```python
from build123d import *

# Parameters (mm, degrees)
SKETCH1_W           = 120
SKETCH1_H           = 30
BOSS_EXTRUDE1_DEPTH = 3
SKETCH2_W           = 28.5
SKETCH2_H           = 30
SKETCH2_W_2         = 20.5
SKETCH2_H_2         = 20.5
BOSS_EXTRUDE2_DEPTH = 20
CHAMFER1_SIZE       = 3
CHAMFER2_SIZE       = 3
CUT_EXTRUDE1_DEPTH  = 20
SKETCH4_R           = 1.65
CUT_EXTRUDE2_DEPTH  = 40
CUT_EXTRUDE3_DEPTH  = 40
SKETCH6_W           = 45.75
SKETCH6_H           = 2
BOSS_EXTRUDE3_DEPTH = 17
CUT_EXTRUDE5_DEPTH  = 17
SKETCH8_R           = 3.302
CUT_EXTRUDE6_DEPTH  = 17
FILLET1_R           = 5


with BuildPart() as part:
    # Sketch1 → Boss-Extrude1 (new body)
    with BuildSketch(Plane(origin=(0, 0, 0), x_dir=(1, 0, 0), z_dir=(0, 1, 0))):
        Rectangle(SKETCH1_W, SKETCH1_H)
    extrude(amount=BOSS_EXTRUDE1_DEPTH)

    # Sketch2 → Boss-Extrude2 (add)
    with BuildSketch(Plane(origin=(0, 3, 0), x_dir=(1, 0, 0), z_dir=(0, 1, 0))):
        Rectangle(SKETCH2_W, SKETCH2_H)
        Rectangle(SKETCH2_W_2, SKETCH2_H_2, mode=Mode.SUBTRACT)
    extrude(amount=BOSS_EXTRUDE2_DEPTH)

    # Chamfer1
    chamfer1_edges = [part.edges().sort_by_distance(p)[0] for p in [
        (14.25, 13, 15),
        (14.25, 13, -15),
        (-14.25, 13, -15),
        (-14.25, 13, 15),
    ]]
    chamfer(chamfer1_edges, length=CHAMFER1_SIZE)

    # Chamfer2
    # the kernel refuses this chamfer: 3 mm, written as the material it takes off along each edge
    with BuildSketch(Plane(origin=(18.965048964, 23, -15), x_dir=(0, -0.9996219169112968, -0.02749587661058619), z_dir=(-1, 0, 0)), Plane(origin=(-18.965048964, 23, 15), x_dir=(0, -0.9996219169112968, 0.02749587661058619), z_dir=(1, 0, 0))) as chamfer2_piece_1:
        Polygon((CHAMFER2_SIZE * 0.999621916911, CHAMFER2_SIZE * 0.0274958766106), (-CHAMFER2_SIZE * 0.0274958766106, CHAMFER2_SIZE * 0.999621916911), (0, 0), align=None)
    extrude(amount=37.930097928, mode=Mode.SUBTRACT)
    with BuildSketch(Plane(origin=(14.25, 23, 19.715048964), x_dir=(0.02749587661058619, -0.9996219169112968, 0), z_dir=(0, 0, -1)), Plane(origin=(-14.25, 23, -19.715048964), x_dir=(-0.02749587661058619, -0.9996219169112968, 0), z_dir=(0, 0, 1))) as chamfer2_piece_2:
        Polygon((CHAMFER2_SIZE * 0.999621916911, CHAMFER2_SIZE * 0.0274958766106), (-CHAMFER2_SIZE * 0.0274958766106, CHAMFER2_SIZE * 0.999621916911), (0, 0), align=None)
    extrude(amount=39.430097928, mode=Mode.SUBTRACT)

    # Sketch3 → Cut-Extrude1 (cut)
    with BuildSketch(Plane(origin=(0, 3, 0), x_dir=(1, 0, 0), z_dir=(0, 1, 0))):
        Polygon((-11.25, 15), (-60, 8), (-60, 15), align=None)
        Polygon((-11.25, -15), (-60, -8), (-60, -15), align=None)
        Polygon((11.25, 15), (60, 15), (60, 8), align=None)
        Polygon((11.25, -15), (60, -15), (60, -8), align=None)
    extrude(amount=-CUT_EXTRUDE1_DEPTH, mode=Mode.SUBTRACT)

    # Sketch4 → Cut-Extrude2 (cut)
    with BuildSketch(Plane.XY.offset(15)):
        with Locations((0, 10.735706987)):
            Circle(SKETCH4_R)
    extrude(amount=-CUT_EXTRUDE2_DEPTH, mode=Mode.SUBTRACT)

    # Sketch5 → Cut-Extrude3 (cut)
    with BuildSketch(Plane(origin=(0, 3, 0), x_dir=(1, 0, 0), z_dir=(0, 1, 0))):
        with BuildLine():
            Line((-9, -1), (-5.916079783, -1))
            ThreePointArc((-5.916079783, -1), (-4.242640687, -4.242640687), (-1, -5.916079783))
            Line((-1, -5.916079783), (-1, -9))
            Line((-1, -9), (1, -9))
            Line((1, -9), (1, -5.916079783))
            ThreePointArc((1, -5.916079783), (4.242640687, -4.242640687), (5.916079783, -1))
            Line((5.916079783, -1), (9, -1))
            Line((9, -1), (9, 1))
            Line((9, 1), (5.916079783, 1))
            ThreePointArc((5.916079783, 1), (4.242640687, 4.242640687), (1, 5.916079783))
            Line((1, 5.916079783), (1, 9))
            Line((1, 9), (-1, 9))
            Line((-1, 9), (-1, 5.916079783))
            ThreePointArc((-1, 5.916079783), (-4.242640687, 4.242640687), (-5.916079783, 1))
            Line((-5.916079783, 1), (-9, 1))
            Line((-9, 1), (-9, -1))
        make_face()
    extrude(amount=-CUT_EXTRUDE3_DEPTH, mode=Mode.SUBTRACT)

    # Sketch6 → Boss-Extrude3 (add)
    with BuildSketch(Plane(origin=(0, 3, 0), x_dir=(1, 0, 0), z_dir=(0, 1, 0))):
        with Locations((-37.125, 0.087113991)):
            Rectangle(SKETCH6_W, SKETCH6_H)
        with Locations((37.125, 0.087113991)):
            Rectangle(SKETCH6_W, SKETCH6_H)
    extrude(amount=BOSS_EXTRUDE3_DEPTH)

    # Sketch7 → Cut-Extrude5 (cut)
    with BuildSketch(Plane.XY.offset(0.912886009)):
        Polygon((-14.25, 20), (-60, 3), (-66.007429388, 26.966086251), align=None)
        Polygon((14.25, 20), (60, 3), (71.057586423, 29.350453949), align=None)
    extrude(amount=-CUT_EXTRUDE5_DEPTH, mode=Mode.SUBTRACT)

    # Sketch8 → Cut-Extrude6 (cut)
    with BuildSketch(Plane.XY.offset(0.912886009)):
        with Locations((-29.25, 8.622465364)):
            Circle(SKETCH8_R)
        with Locations((29.25, 8.622465364)):
            Circle(SKETCH8_R)
    extrude(amount=-CUT_EXTRUDE6_DEPTH, mode=Mode.SUBTRACT)

    # Fillet1
    fillet1_edges = [part.edges().sort_by_distance(p)[0] for p in [
        (-60, 1.5, -8),
        (-60, 1.5, 8),
        (60, 1.5, -8),
        (60, 1.5, 8),
    ]]
    fillet(fillet1_edges, radius=FILLET1_R)


solid = part.part
```
Here's how the part is built. I have some questions about the finished solid (model axes, mm). A direction names the side the tool comes from. Round coordinates to 2 decimals unless told otherwise and drop trailing zeros. Order: outer loops, then holes, each group sorted by start corner. A loop starts at its lowest first (then second) coordinate and runs counter-clockwise, first axis right, second up. Notation, with made-up numbers: (17.5, -14.5) -> (55.5, -14.5) arc R21 ccw to (55.5, 2.5) -> close; hole circle Ø5 at (65, 56.5). An arc over 180 degrees is marked (long way). Use a Markdown table: item, result. Add a question column.
(1) Suppose I cut it at C-C, the plane x = -3.5. Please give me the cut outline in (y, z), and give its area (3 significant figures).
(2) I need wall thicknesses on line 1 along X through (y, z) = (10.5, -2.5); line 2 along Y through (x, z) = (0, 11.8); line 3 along Y through (x, z) = (-19.5, -5.5). Which ranges of each line are inside material? Lowest first, please.
(3) Suppose I cut it at D-D, the plane x = -24.5. Please give me the cut outline in (y, z).
(4) Suppose I cut it at B-B, the plane y = 16. Please give me the cut outline in (x, z).
(5) If we mould it in two halves opening along X, with no side actions, what happens to faces 1 (the face through (12.77, 12.12, -13.48)), 2 (the face through (0, 2, -9)), 3 (the face through (-1, 23, 11))? For each: released by +X, released by -X, zero draft, split by the parting line, or undercut.
(6) For pin 1 Ø3 at (x, z) = (47, -1) entering from -Y; pin 2 Ø2 at (x, y) = (-29, 17) entering from +Z; pin 3 Ø6 at (y, z) = (12, -5) entering from -X; pin 4 Ø13.5 at (x, y) = (-38, 15) entering from -Z, each with a flat end and sliding along its axis, tell me the tip position at first contact or that it passes through.
(7) For faces 4 (the face through (35, 3, -7)), 5 (the face through (-10.25, 13, 0)), 6 (the face through (9, 2, 0)), 7 (the face through (35, 3, 6)), which set-ups out of +Z, -Z, +X, -X, +Y, -Y let a thin tool reach every point of the face, with its end or its side?
(8) Suppose I cut it at A-A, the plane y = 7.25. Please give me the cut outline in (x, z), and give its area (3 significant figures).
Verdict:
| question | item | result |
|---|---|---|
| 1 | outline | (0, -15) -> (20, -15) -> (23, -12) -> (23, -10.25) -> (3, -10.25) -> (3, -4.87) -> (0, -4.87) -> close; (0, 4.87) -> (3, 4.87) -> (3, 10.25) -> (23, 10.25) -> (23, 12) -> (20, 15) -> (0, 15) -> close |
| 1 | area | 242 mm2 |
| 2 | line 1 | -14.25 to -10.25, 10.25 to 14.25 |
| 2 | line 2 | 0 to 9.09, 12.39 to 23 |
| 2 | line 3 | 0 to 3 |
| 3 | outline | (0, -13.1) -> (3, -13.1) -> (3, -1.09) -> (16.19, -1.09) -> (16.19, 0.91) -> (3, 0.91) -> (3, 13.1) -> (0, 13.1) -> close |
| 4 | outline | (-25.01, -1.09) -> (-14.25, -1.09) -> (-14.25, -12) -> (-11.25, -15) -> (11.25, -15) -> (14.25, -12) -> (14.25, -1.09) -> (25.01, -1.09) -> (25.01, 0.91) -> (14.25, 0.91) -> (14.25, 12) -> (11.25, 15) -> (-11.25, 15) -> (-14.25, 12) -> (-14.25, 0.91) -> (-25.01, 0.91) -> close; hole (-10.25, -10.25) -> (10.25, -10.25) -> (10.25, 10.25) -> (-10.25, 10.25) -> close |
| 5 | face 1 | released by +X |
| 5 | face 2 | undercut |
| 5 | face 3 | zero draft |
| 6 | pin 1 | y = 0 |
| 6 | pin 2 | through |
| 6 | pin 3 | x = -14.25 |
| 6 | pin 4 | z = -1.09 |
| 7 | face 4 | -Z, +X, +Y |
| 7 | face 5 | +Y |
| 7 | face 6 | +Y, -Y |
| 7 | face 7 | +Z, +X, +Y |
| 8 | outline | (-48.56, -1.09) -> (-32.25, -1.09) -> (-32.25, 0.91) -> (-48.56, 0.91) -> close; (-26.25, -1.09) -> (-14.25, -1.09) -> (-14.25, -12) -> (-11.25, -15) -> (11.25, -15) -> (14.25, -12) -> (14.25, -1.09) -> (26.25, -1.09) -> (26.25, 0.91) -> (14.25, 0.91) -> (14.25, 12) -> (11.25, 15) -> (-11.25, 15) -> (-14.25, 12) -> (-14.25, 0.91) -> (-26.25, 0.91) -> close; (32.25, -1.09) -> (48.56, -1.09) -> (48.56, 0.91) -> (32.25, 0.91) -> close; hole (-10.25, -10.25) -> (10.25, -10.25) -> (10.25, 10.25) -> (-10.25, 10.25) -> close |
| 8 | area | 530 mm2 |
